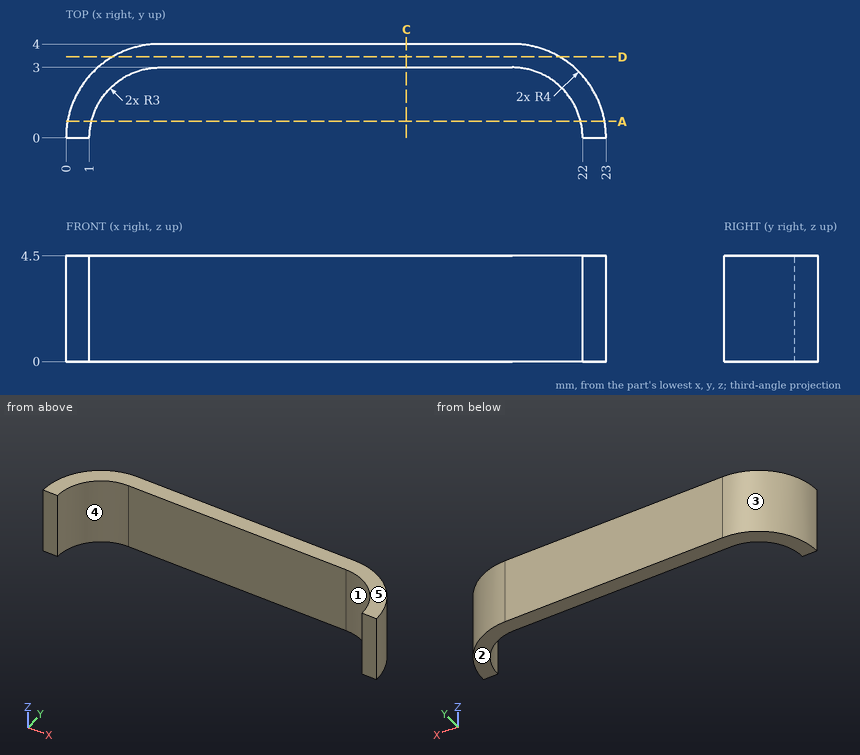
Job drawing, mm, ordinate dimensions from the low corner. One solid piece. A direction names the side the tool comes from. Coordinates: 2 decimals unless noted, no trailing zeros. Order: outer loops, then holes, each group sorted by start corner. A loop starts at its lowest first (then second) coordinate and runs counter-clockwise, first axis right, second up. Notation, with made-up numbers: (14.5, 16.5) -> (34.5, 16.5) arc R23 ccw to (34.5, 30.5) -> close; hole circle Ø1 at (60.25, 50). An arc over 180 degrees is marked (long way). Answer in a Markdown table with one row per item. Add a question column.
Q1. Band-saw the part on D-D, the plane y = 3.45. List the corners of the cut face in (x, z), then the cut area to 3 significant figures.
Q2. Band-saw the part on A-A, the plane y = 0.7. List the corners of the cut face in (x, z), then the cut area to 3 significant figures.
Q3. Which spindle directions (+Z, -Z, +X, -X, +Y, -Y) get a long thin tool onto all of the face, cutting with end or side? Do the marked faces 4 and 5. Say none if no direction does.
Q4. Band-saw the part on C-C, the plane x = 14.5. List the corners of the cut face in (y, z), then the cut area to 3 significant figures.
Q5. Mould opens along X. For the marked faces 1, 2 and 3 say: +X half, -X half, draft (parallel to the pull), parting line (faces both ways), or undercut.
Q6. Drop a flat-ended pin along its axis: pin 1 (2 mm diameter, centred on x = 6, z = 1, fed in from -Y). Give the stop position or say it passes through.
Q7. Wall check: line 1 along Y through (x, z) = (4.75, 0.9); line 2 along X through (y, z) = (2.3, 0.9); line 3 along X through (y, z) = (1.5, 0.8). Give the ranges that are in metal, low to high. Write a range as [from, to].
Answers follow:
| question | item | result |
|---|---|---|
| 1 | outline | (1.98, 0) -> (21.02, 0) -> (21.02, 4.5) -> (1.98, 4.5) -> close |
| 1 | area | 85.7 mm^2 |
| 2 | outline | (0.06, 0) -> (1.08, 0) -> (1.08, 4.5) -> (0.06, 4.5) -> close; (21.92, 0) -> (22.94, 0) -> (22.94, 4.5) -> (21.92, 4.5) -> close |
| 2 | area | 9.19 mm^2 |
| 3 | face 4 | +Z, -Z, -Y |
| 3 | face 5 | +Z, +X, -X, +Y, -Y |
| 4 | outline | (3, 0) -> (4, 0) -> (4, 4.5) -> (3, 4.5) -> close |
| 4 | area | 4.50 mm^2 |
| 5 | face 1 | undercut |
| 5 | face 2 | draft |
| 5 | face 3 | -X half |
| 6 | pin 1 | y = 3 |
| 7 | line 1 | [3, 4] |
| 7 | line 2 | [0.73, 2.07], [20.93, 22.27] |
| 7 | line 3 | [0.29, 1.4], [21.6, 22.71] |
